```python
from build123d import *

# Parameters (mm, degrees)
SKETCH_1_R          = 1.55
SKETCH_1_R_2        = 10
SKETCH_1_R_3        = 1.6
EXTRUDE_1_DEPTH     = 2
CUT_EXTRUDE_1_DEPTH = 10


with BuildPart() as part:
    # 草图1 → 凸台-拉伸1 (new body)
    with BuildSketch(Plane.XZ):
        with BuildLine():
            Line((-70, -100), (70, -100))
            ThreePointArc((70, -100), (77.071067812, -97.071067812), (80, -90))
            Line((80, -90), (80, 90))
            ThreePointArc((80, 90), (77.071067812, 97.071067812), (70, 100))
            Line((70, 100), (-70, 100))
            ThreePointArc((-70, 100), (-77.071067812, 97.071067812), (-80, 90))
            Line((-80, 90), (-80, -90))
            ThreePointArc((-80, -90), (-77.071067812, -97.071067812), (-70, -100))
        make_face()
        with Locations(Location((0, 50.5527, 0), (0, 0, 90))):
            Circle(SKETCH_1_R, mode=Mode.SUBTRACT)
        with Locations(Location((0, 57.5527, 0), (0, 0, 90))):
            Circle(SKETCH_1_R, mode=Mode.SUBTRACT)
        with Locations(Location((0, 64.5527, 0), (0, 0, 90))):
            Circle(SKETCH_1_R, mode=Mode.SUBTRACT)
        with Locations(Location((0, 71.5527, 0), (0, 0, 90))):
            Circle(SKETCH_1_R, mode=Mode.SUBTRACT)
        with Locations(Location((0, 78.5527, 0), (0, 0, 90))):
            Circle(SKETCH_1_R, mode=Mode.SUBTRACT)
        with Locations(Location((0, 85.5527, 0), (0, 0, 90))):
            Circle(SKETCH_1_R, mode=Mode.SUBTRACT)
        with Locations(Location((-30, 30, 0), (0, 0, 90))):
            Circle(SKETCH_1_R_2, mode=Mode.SUBTRACT)
        with Locations(Location((30, 30, 0), (0, 0, 90))):
            Circle(SKETCH_1_R_2, mode=Mode.SUBTRACT)
        with Locations(Location((55, 75, 0), (0, 0, 90))):
            Circle(SKETCH_1_R_3, mode=Mode.SUBTRACT)
        with Locations(Location((55, 0, 0), (0, 0, 90))):
            Circle(SKETCH_1_R_3, mode=Mode.SUBTRACT)
        with Locations(Location((55, -75, 0), (0, 0, 90))):
            Circle(SKETCH_1_R_3, mode=Mode.SUBTRACT)
        with Locations(Location((-55, -75, 0), (0, 0, 90))):
            Circle(SKETCH_1_R_3, mode=Mode.SUBTRACT)
        with Locations(Location((-55, 0, 0), (0, 0, 90))):
            Circle(SKETCH_1_R_3, mode=Mode.SUBTRACT)
        with Locations(Location((-55, 75, 0), (0, 0, 90))):
            Circle(SKETCH_1_R_3, mode=Mode.SUBTRACT)
        with BuildLine():
            Line((37.5, -1.55), (7.5, -1.55))
            ThreePointArc((7.5, -1.55), (5.95, 0), (7.5, 1.55))
            Line((7.5, 1.55), (35.95, 1.55))
            Line((35.95, 1.55), (35.95, 16))
            ThreePointArc((35.95, 16), (37.5, 17.55), (39.05, 16))
            Line((39.05, 16), (39.05, 0))
            ThreePointArc((39.05, 0), (38.596015511, -1.096015511), (37.5, -1.55))
        make_face(mode=Mode.SUBTRACT)
        with BuildLine():
            Line((-35.95, 1.55), (-35.95, 16))
            ThreePointArc((-35.95, 16), (-37.5, 17.55), (-39.05, 16))
            Line((-39.05, 16), (-39.05, 0))
            ThreePointArc((-39.05, 0), (-38.596015511, -1.096015511), (-37.5, -1.55))
            Line((-37.5, -1.55), (-7.5, -1.55))
            ThreePointArc((-7.5, -1.55), (-5.95, 0), (-7.5, 1.55))
            Line((-7.5, 1.55), (-35.95, 1.55))
        make_face(mode=Mode.SUBTRACT)
        with BuildLine():
            Line((39.05, -66), (39.05, -17.55))
            ThreePointArc((39.05, -17.55), (37.5, -16), (35.95, -17.55))
            Line((35.95, -17.55), (35.95, -66))
            ThreePointArc((35.95, -66), (37.5, -67.55), (39.05, -66))
        make_face(mode=Mode.SUBTRACT)
        with BuildLine():
            Line((-35.95, -17.55), (-35.95, -66))
            ThreePointArc((-35.95, -66), (-37.5, -67.55), (-39.05, -66))
            Line((-39.05, -66), (-39.05, -17.55))
            ThreePointArc((-39.05, -17.55), (-37.5, -16), (-35.95, -17.55))
        make_face(mode=Mode.SUBTRACT)
        with BuildLine():
            Line((8, -83.55), (-8, -83.55))
            ThreePointArc((-8, -83.55), (-16, -75.55), (-8, -67.55))
            Line((-8, -67.55), (8, -67.55))
            ThreePointArc((8, -67.55), (16, -75.55), (8, -83.55))
        make_face(mode=Mode.SUBTRACT)
        with BuildLine():
            Line((8.55, 85.5527), (8.55, 50.5527))
            ThreePointArc((8.55, 50.5527), (7, 49.0027), (5.45, 50.5527))
            Line((5.45, 50.5527), (5.45, 85.5527))
            ThreePointArc((5.45, 85.5527), (7, 87.1027), (8.55, 85.5527))
        make_face(mode=Mode.SUBTRACT)
        with BuildLine():
            Line((-8.55, 50.5527), (-8.55, 85.5527))
            ThreePointArc((-8.55, 85.5527), (-7, 87.1027), (-5.45, 85.5527))
            Line((-5.45, 85.5527), (-5.45, 50.5527))
            ThreePointArc((-5.45, 50.5527), (-7, 49.0027), (-8.55, 50.5527))
        make_face(mode=Mode.SUBTRACT)
        with BuildLine():
            Line((42, 93.45), (21, 93.45))
            ThreePointArc((21, 93.45), (19.45, 95), (21, 96.55))
            Line((21, 96.55), (42, 96.55))
            ThreePointArc((42, 96.55), (43.55, 95), (42, 93.45))
        make_face(mode=Mode.SUBTRACT)
        with BuildLine():
            Line((-21, 93.45), (-42, 93.45))
            ThreePointArc((-42, 93.45), (-43.55, 95), (-42, 96.55))
            Line((-42, 96.55), (-21, 96.55))
            ThreePointArc((-21, 96.55), (-19.45, 95), (-21, 93.45))
        make_face(mode=Mode.SUBTRACT)
        with BuildLine():
            Line((14, 93.45), (-14, 93.45))
            ThreePointArc((-14, 93.45), (-15.55, 95), (-14, 96.55))
            Line((-14, 96.55), (14, 96.55))
            ThreePointArc((14, 96.55), (15.55, 95), (14, 93.45))
        make_face(mode=Mode.SUBTRACT)
        with BuildLine():
            Line((21, -93.45), (42, -93.45))
            ThreePointArc((42, -93.45), (43.55, -95), (42, -96.55))
            Line((42, -96.55), (21, -96.55))
            ThreePointArc((21, -96.55), (19.45, -95), (21, -93.45))
        make_face(mode=Mode.SUBTRACT)
        with BuildLine():
            Line((-42, -93.45), (-21, -93.45))
            ThreePointArc((-21, -93.45), (-19.45, -95), (-21, -96.55))
            Line((-21, -96.55), (-42, -96.55))
            ThreePointArc((-42, -96.55), (-43.55, -95), (-42, -93.45))
        make_face(mode=Mode.SUBTRACT)
        with BuildLine():
            Line((-14, -93.45), (14, -93.45))
            ThreePointArc((14, -93.45), (15.55, -95), (14, -96.55))
            Line((14, -96.55), (-14, -96.55))
            ThreePointArc((-14, -96.55), (-15.55, -95), (-14, -93.45))
        make_face(mode=Mode.SUBTRACT)
    extrude(amount=-EXTRUDE_1_DEPTH)

    # 草图2 → 切除-拉伸1 (cut)
    with BuildSketch(Plane.XZ):
        with BuildLine():
            Line((-17, -17.275), (-17, -29.275))
            ThreePointArc((-17, -29.275), (-18.5, -30.775), (-20, -29.275))
            Line((-20, -29.275), (-20, -17.275))
            ThreePointArc((-20, -17.275), (-18.5, -15.775), (-17, -17.275))
        make_face()
        with BuildLine():
            Line((-17, -54.275), (-17, -66.275))
            ThreePointArc((-17, -66.275), (-18.5, -67.775), (-20, -66.275))
            Line((-20, -66.275), (-20, -54.275))
            ThreePointArc((-20, -54.275), (-18.5, -52.775), (-17, -54.275))
        make_face()
        with BuildLine():
            Line((17, -54.275), (17, -66.275))
            ThreePointArc((17, -66.275), (18.5, -67.775), (20, -66.275))
            Line((20, -66.275), (20, -54.275))
            ThreePointArc((20, -54.275), (18.5, -52.775), (17, -54.275))
        make_face()
        with BuildLine():
            Line((17, -17.275), (17, -29.275))
            ThreePointArc((17, -29.275), (18.5, -30.775), (20, -29.275))
            Line((20, -29.275), (20, -17.275))
            ThreePointArc((20, -17.275), (18.5, -15.775), (17, -17.275))
        make_face()
    extrude(amount=-CUT_EXTRUDE_1_DEPTH, mode=Mode.SUBTRACT)


solid = part.part
```
Here's how the part is built. I have some questions about the finished solid (model axes, mm). A direction names the side the tool comes from. Coordinates: 2 decimals unless noted, no trailing zeros. Order: outer loops, then holes, each group sorted by start corner. A loop starts at its lowest first (then second) coordinate and runs counter-clockwise, first axis right, second up.
Item 1: If we section it at A-A, the plane x = -30: List the corners of the cut face in (y, z) for me, then the cut area to 3 significant figures.
Response values:
outline: (0, -100) - (2, -100) - (2, -96.55) - (0, -96.55) - close; (0, -93.45) - (2, -93.45) - (2, -1.55) - (0, -1.55) - close; (0, 1.55) - (2, 1.55) - (2, 20) - (0, 20) - close; (0, 40) - (2, 40) - (2, 93.45) - (0, 93.45) - close; (0, 96.55) - (2, 96.55) - (2, 100) - (0, 100) - close
area: 341 mm2
Item 2: If we section it at C-C, the plane y = 1.45: Give the number of separate pieces and of enclosed holes in the cut face, then the cut area to 3 significant figures.
Response values:
separate pieces: 1
enclosed holes: 31
area: 29,200 mm2
Item 3: I need wall thicknesses on probe 1 along Z at (x, y) = (5, 0.25); probe 2 along Z at (x, y) = (-55, 0.45); probe 3 along X at (y, z) = (0.7, 13). Which ranges of each line are inside material? Lowest first, please.
Response values:
probe 1: z = -100 to -96.55, -93.45 to -83.55, -67.55 to 93.45, 96.55 to 100
probe 2: z = -100 to -76.6, -73.4 to -1.6, 1.6 to 73.4, 76.6 to 100
probe 3: x = -80 to -39.05, -35.95 to 35.95, 39.05 to 80
Item 4: Thinking about a two-plate mould opening in X: for faces 1 (the face through (76.99, 0.99, -97.15)), 2 (the face through (-1, 2, 1)), 3 (the face through (16, 1, -75.4)), which applies, pulls with the +X half, pulls with the -X half, needs draft (parallel to the pull), parting line crosses it, or undercut?
Response values:
face 1: pulls with the +X half
face 2: needs draft
face 3: undercut
Item 5: If we section it at B-B, the plane z = -35: List the corners of the cut face in (x, y) for me, then the cut area to 3 significant figures.
Response values:
outline: (-80, 0) - (-39.05, 0) - (-39.05, 2) - (-80, 2) - close; (-35.95, 0) - (35.95, 0) - (35.95, 2) - (-35.95, 2) - close; (39.05, 0) - (80, 0) - (80, 2) - (39.05, 2) - close
area: 308 mm2
Item 6: Which directions (+Z, -Z, +X, -X, +Y, -Y) give clear straight access to the entire face, cutting with the end or side of a thin tool? Please do faces 4 (the face through (-16, 1, -75.7)), 5 (the face through (-1, 0, 1)).
Response values:
face 4: +Y, -Y
face 5: +Z, -Z, +X, -X, -Y
